Here's how the part is built. I have some questions about the finished solid (model axes, mm). Give positions to 0.01 mm unless a question says otherwise; leave off trailing zeros. Order: outer loops, then holes, each group sorted by start corner. A loop starts at its lowest first (then second) coordinate and runs counter-clockwise, first axis right, second up. Notation, with made-up numbers: (-26, -11) -> (-2, -11) arc R24 ccw to (-2, 5) -> close; hole circle Ø5 at (-8, 52.25). An arc over 180 degrees is marked (long way). Write each question's results on one line, items separated by ' | '. Start each with the question number.
Q1. I'm going to push flat-ended pins straight in: pin 1 (1 mm diameter, centred on x = 1.5, y = 1.5, fed in from +Z); pin 2 (2 mm diameter, centred on x = -3, z = 2.5, fed in from +Y); pin 3 (1.5 mm diameter, centred on x = -1, y = -3.5, fed in from +Z). Where does each tip first touch, or does it pass through?
Q2. I need wall thicknesses on line 1 along Z through (x, y) = (2.5, -3.25); line 2 along Y through (x, z) = (0, 0.25); line 3 along Y through (x, z) = (0, 1). Which ranges of each line are inside material? Lowest first, please. Write a range as [from, to].
Q3. Imagine slicing it at B-B, the plane z = -0.5. Please give me the cut outline in (x, y), then the cut area to 3 significant figures.
Q4. Imagine slicing it at A-A, the plane z = 1.5. Please give me the cut outline in (x, y).
```python
from build123d import *

# Parameters (mm, degrees)
F2_R          = 1.5
F3_DEPTH      = 3.998497265
F3_DEPTH_BACK = 4.0006311494


with BuildPart() as f1:
    # F0 (on Front) → F1 (revolve)
    with BuildSketch(Plane.XZ):
        with BuildLine():
            Line((-3.878140574, -1.9962841181), (-3.4647271293, -1.9964134512))
            ThreePointArc((-3.4647271293, -1.9964134512), (-2.0005418335, -3.4612859959), (0, -3.997497265))
            Line((0, -3.997497265), (0, 3.9996311494))
            ThreePointArc((0, 3.9996311494), (-2.000079858, 3.4636866573), (-3.4641938241, 1.9994714302))
            Line((-3.4641938241, 1.9994714302), (-3.9530518044, 1.9994488908))
            ThreePointArc((-3.9530518044, 1.9994488908), (-5.9981910715, 0.0850437646), (-4.1231084445, -1.9962074819))
            Line((-4.1231084445, -1.9962074819), (-3.878140574, -1.9962841181))
        make_face()
        with BuildLine():
            ThreePointArc((-4.1231084445, -1.9962074819), (-4.0006256837, -1.9999999021), (-3.878140574, -1.9962841181))
            Line((-3.878140574, -1.9962841181), (-4.1231084445, -1.9962074819))
        make_face()
    revolve(axis=Axis((0, 0, 0.0010669422), (0, 0, -1)))

    # F2 (on Top) → F3 (cut, two sides)
    with BuildSketch(Plane.XY) as f3_sk:
        Circle(F2_R)
    extrude(amount=-F3_DEPTH, mode=Mode.SUBTRACT)
    extrude(f3_sk.sketch, amount=F3_DEPTH_BACK, mode=Mode.SUBTRACT)


solid = f1.part
```
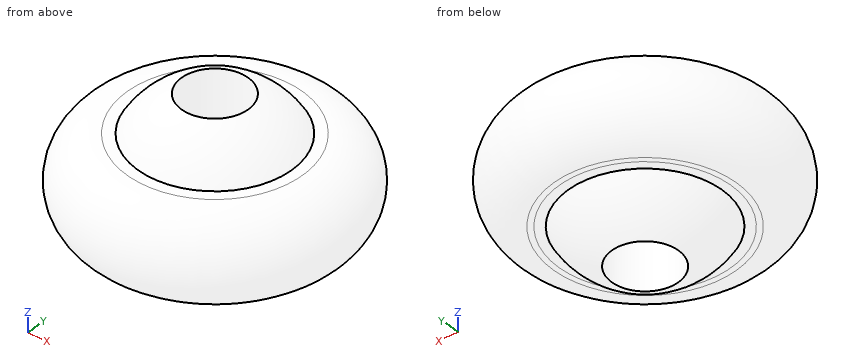
Geometry check:
1) pin 1: z = 3.66 | pin 2: y = 4.53 | pin 3: z = 2.77
2) line 1: [-2, 2] | line 2: [-5.98, -1.5], [1.5, 5.98] | line 3: [-5.73, -1.5], [1.5, 5.73]
3) outline: circle Ø11.87 at (0, 0); hole circle Ø3 at (0, 0) | area: 104 mm²
4) outline: circle Ø10.65 at (0, 0); hole circle Ø3 at (0, 0)
